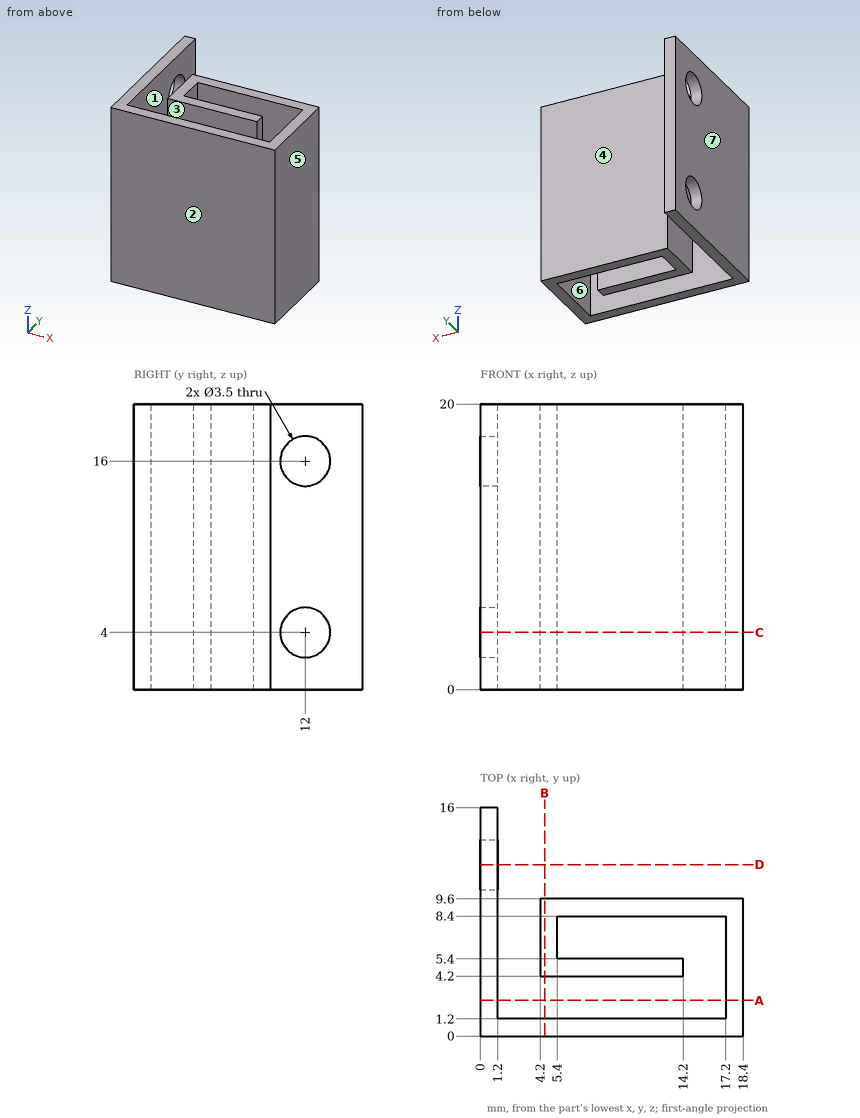
Could you check a few things on this drawing? It's one solid part, dimensions in mm from its lowest x, y, z. A direction names the side the tool comes from. Round coordinates to 2 decimals unless told otherwise and drop trailing zeros. Loops run counter-clockwise (first coordinate to the right, second up) from the corner with the lowest first, then second, coordinate; pieces in that order, holes last. Notation, with made-up numbers: (-0.75, 55) -> (22.25, 55) arc R11 cw to (22.25, 59) -> close; hole circle Ø10 at (-33, 72). An arc over 180 degrees is marked (long way). One line per item, written item: value. Start each with the question number.
1. If I drill on probe 1 along Y at (x, z) = (7.5, 4.5); probe 2 along X at (y, z) = (4.25, 13.5); probe 3 along Y at (x, z) = (4.75, 15), over which ranges is the centre line in solid material (lowest first)?
2. If we section it at D-D, the plane y = 12: Write out the boundary of the cut face in (x, z).
3. If we section it at B-B, the plane x = 4.5: Write out the boundary of the cut face in (y, z).
4. For pin 1 (7 mm diameter, centred on x = 9, z = 13, fed in from +Y); pin 2 (8 mm diameter, centred on x = 10.5, z = 13.5, fed in from -Y), each with a flat end and sliding along its axis, tell me the tip position at first contact or that it passes through.
5. For the marked faces 1, 2 and 3, which set-ups out of +Z, -Z, +X, -X, +Y, -Y let a thin tool reach every point of the face, with its end or its side?
6. If we section it at A-A, the plane y = 2.5: Write out the boundary of the cut face in (x, z), then the cut area to 3 significant figures.
7. If we mould it in two halves opening along X, with no side actions, what happens to the marked faces 4, 5, 6 and 7? For each: pulls with the +X half, pulls with the -X half, needs draft (parallel to the pull), parting line crosses it, or undercut.
8. If we section it at C-C, the plane z = 4: Write out the boundary of the cut face in (x, y).
Calculated:
1. probe 1: y = 0 to 1.2, 4.2 to 5.4, 8.4 to 9.6
1. probe 2: x = 0 to 1.2, 4.2 to 14.2, 17.2 to 18.4
1. probe 3: y = 0 to 1.2, 4.2 to 9.6
2. outline: (0, 0) -> (1.2, 0) -> (1.2, 2.25) -> (0, 2.25) -> close; (0, 5.75) -> (1.2, 5.75) -> (1.2, 14.25) -> (0, 14.25) -> close; (0, 17.75) -> (1.2, 17.75) -> (1.2, 20) -> (0, 20) -> close
3. outline: (0, 0) -> (1.2, 0) -> (1.2, 20) -> (0, 20) -> close; (4.2, 0) -> (9.6, 0) -> (9.6, 20) -> (4.2, 20) -> close
4. pin 1: stops at y = 9.6
4. pin 2: stops at y = 0
5. face 1: +Z, -Z, +Y
5. face 2: +Z, -Z, +X, -X, -Y
5. face 3: +Z, -Z
6. outline: (0, 0) -> (1.2, 0) -> (1.2, 20) -> (0, 20) -> close; (17.2, 0) -> (18.4, 0) -> (18.4, 20) -> (17.2, 20) -> close
6. area: 48.0 mm²
7. face 4: needs draft
7. face 5: pulls with the +X half
7. face 6: undercut
7. face 7: pulls with the -X half
8. outline: (0, 0) -> (18.4, 0) -> (18.4, 9.6) -> (4.2, 9.6) -> (4.2, 4.2) -> (14.2, 4.2) -> (14.2, 5.4) -> (5.4, 5.4) -> (5.4, 8.4) -> (17.2, 8.4) -> (17.2, 1.2) -> (1.2, 1.2) -> (1.2, 10.25) -> (0, 10.25) -> close; (0, 13.75) -> (1.2, 13.75) -> (1.2, 16) -> (0, 16) -> close
